from build123d import *

# Parameters (mm, degrees)
F0_W      = 23.4
F0_H      = 7.4
F1_DEPTH  = 3.95
F2_R      = 3.69999
F3_R      = 2.499
F4_DEPTH  = 25
F3_R_2    = 3
F5_DEPTH  = 1
F6_R      = 3
F6_R_2    = 2.499
F7_DEPTH  = 1
F8_R      = 3
F9_DEPTH  = 0.5
F10_R     = 3
F11_DEPTH = 0.5


# Not quite as in the source:
# - a fillet or chamfer is up to 0.001 mm smaller than in the source, because OpenCascade refuses the exact size


with BuildPart() as f1:
    # F0 (on Front) → F1 (new body, symmetric)
    with BuildSketch(Plane.XZ):
        Rectangle(F0_W, F0_H)
        with BuildLine():
            ThreePointArc((-7.199, -2.3313088598), (-8.099, -2.499), (-8.999, -2.3313088598))
            Line((-8.999, -2.3313088598), (-8.999, -0.9))
            Line((-8.999, -0.9), (-10.4303088598, -0.9))
            ThreePointArc((-10.4303088598, -0.9), (-10.598, 0), (-10.4303088598, 0.9))
            Line((-10.4303088598, 0.9), (-8.999, 0.9))
            Line((-8.999, 0.9), (-8.999, 2.3313088598))
            ThreePointArc((-8.999, 2.3313088598), (-8.099, 2.499), (-7.199, 2.3313088598))
            Line((-7.199, 2.3313088598), (-7.199, 0.9))
            Line((-7.199, 0.9), (-5.7676911402, 0.9))
            ThreePointArc((-5.7676911402, 0.9), (-5.6, 0), (-5.7676911402, -0.9))
            Line((-5.7676911402, -0.9), (-7.199, -0.9))
            Line((-7.199, -0.9), (-7.199, -2.3313088598))
        make_face(mode=Mode.SUBTRACT)
        with BuildLine():
            Line((7.199, 0.9), (7.199, 2.3313088598))
            ThreePointArc((7.199, 2.3313088598), (8.099, 2.499), (8.999, 2.3313088598))
            Line((8.999, 2.3313088598), (8.999, 0.9))
            Line((8.999, 0.9), (10.4303088598, 0.9))
            ThreePointArc((10.4303088598, 0.9), (10.598, 0), (10.4303088598, -0.9))
            Line((10.4303088598, -0.9), (8.999, -0.9))
            Line((8.999, -0.9), (8.999, -2.3313088598))
            ThreePointArc((8.999, -2.3313088598), (8.099, -2.499), (7.199, -2.3313088598))
            Line((7.199, -2.3313088598), (7.199, -0.9))
            Line((7.199, -0.9), (5.7676911402, -0.9))
            ThreePointArc((5.7676911402, -0.9), (5.6, 0), (5.7676911402, 0.9))
            Line((5.7676911402, 0.9), (7.199, 0.9))
        make_face(mode=Mode.SUBTRACT)
    extrude(amount=F1_DEPTH, both=True)

    # F2 (radius 3.7 in the source; OpenCascade refuses exactly that, so slightly less here)
    f2_edges = [f1.edges().sort_by_distance(p)[0] for p in [
        (-11.7, 0, -3.7),
        (-11.7, 0, 3.7),
        (11.7, 0, 3.7),
        (11.7, 0, -3.7),
    ]]
    fillet(f2_edges, radius=F2_R)

    # F3 (on face) → F4 (cut)
    with BuildSketch(Plane.XY.offset(3.7)):
        Circle(F3_R)
    extrude(amount=-F4_DEPTH, mode=Mode.SUBTRACT)

    # F3 (on face) → F5 (cut)
    with BuildSketch(Plane.XY.offset(3.7)):
        Circle(F3_R_2)
        Circle(F3_R, mode=Mode.SUBTRACT)
    extrude(amount=-F5_DEPTH, mode=Mode.SUBTRACT)

    # F6 (on face) → F7 (cut)
    with BuildSketch(Plane(origin=(0, 0, -3.7), x_dir=(1, 0, 0), z_dir=(0, 0, -1))):
        Circle(F6_R)
        Circle(F6_R_2, mode=Mode.SUBTRACT)
    extrude(amount=-F7_DEPTH, mode=Mode.SUBTRACT)

    # F8 (on face) → F9 (cut)
    with BuildSketch(Plane.XZ.offset(3.95)):
        with Locations((-8, 0)):
            Circle(F8_R)
        with Locations((8.099, 0)):
            Circle(F8_R)
    extrude(amount=-F9_DEPTH, mode=Mode.SUBTRACT)

    # F10 (on face) → F11 (cut)
    with BuildSketch(Plane(origin=(0, 3.95, 0), x_dir=(-1, 0, 0), z_dir=(0, 1, 0))):
        with Locations((-8, 0)):
            Circle(F10_R)
        with Locations((8.099, 0)):
            Circle(F10_R)
    extrude(amount=-F11_DEPTH, mode=Mode.SUBTRACT)


solid = f1.part
Verification items for the finished model (mm, model axes). A direction names the side the tool comes from. Give positions to 0.01 mm unless a question says otherwise; leave off trailing zeros. Order: outer loops, then holes, each group sorted by start corner. A loop starts at its lowest first (then second) coordinate and runs counter-clockwise, first axis right, second up. Notation, with made-up numbers: (-27, -14.75) -> (-16, -14.75) arc R22 ccw to (-16, 8.25) -> close; hole circle Ø10 at (-32, 87). An arc over 180 degrees is marked (long way). Answer as CSV lines item,"result".
Q1. Release check for a two-part mould opening along Y. For faces 4 (the flat face through (-2, 2, 2.7)), 5 (the flat face through (6, 0, -0.9)), 6 (the flat face through (9.4, -3.45, -1.3)), 7 (the cylindrical face through (-3, 0, 3)) record: +Y half, -Y half, draft (parallel to the pull), parting line (faces both ways), or undercut.
Solutions:
face 4,"undercut"
face 5,"draft"
face 6,"-Y half"
face 7,"undercut"
Q2. Sectioned sample at B-B on x = 0. Record the cut outline in (y, z), plus the area to 3 significant figures.
Solutions:
outline,"(-3.95, -3.7) -> (-3, -3.7) -> (-3, -2.7) -> (-2.5, -2.7) -> (-2.5, 2.7) -> (-3, 2.7) -> (-3, 3.7) -> (-3.95, 3.7) -> close; (2.5, -2.7) -> (3, -2.7) -> (3, -3.7) -> (3.95, -3.7) -> (3.95, 3.7) -> (3, 3.7) -> (3, 2.7) -> (2.5, 2.7) -> close"
area,"19.5 mm²"
Q3. Depth check by flat-ended pin: pin 1 (3 mm diameter, centred on y = 2, z = -2, fed in from -X); pin 2 (0.7 mm diameter, centred on y = 1, z = -1.5, fed in from +X); pin 3 (4 mm diameter, centred on x = 0, y = 0, fed in from -Z); pin 4 (4 mm diameter, centred on y = 2.5, z = -3, fed in from +X). Enter the tip coordinate at first touch or a pass-through.
Solutions:
pin 1,"stops at x = -11.67"
pin 2,"stops at x = 11.52"
pin 3,"passes through"
pin 4,"stops at x = 11.56"
Q4. Scan lines: probe 1 along X at (y, z) = (0, 1.15); probe 2 along X at (y, z) = (-2, 2); probe 3 along Z at (x, y) = (-8, -3.75). Record each from-to range of solid material in increasing order.
Solutions:
probe 1,"x = -11.52 to -9, -7.2 to -2.5, 2.5 to 7.2, 9 to 11.52"
probe 2,"x = -11.11 to -9, -7.2 to -1.5, 1.5 to 7.2, 9 to 11.11"
probe 3,"z = -3.7 to -3, 3 to 3.7"
Q5. Sectioned sample at A-A on z = -1.75. Count the separate pieces of the cut face and the enclosed holes in it, plus the area to 3 significant figures.
Solutions:
separate pieces,"3"
enclosed holes,"1"
area,"124 mm²"
Q6. Sectioned sample at D-D on x = 8.5. Record the cut outline in (y, z), plus the area to 3 significant figures.
Solutions:
outline,"(-3.95, -3.67) -> (3.95, -3.67) -> (3.95, -2.96) -> (3.45, -2.96) -> (3.45, -2.47) -> (-3.45, -2.47) -> (-3.45, -2.97) -> (-3.95, -2.97) -> close; (-3.95, 2.97) -> (-3.45, 2.97) -> (-3.45, 2.47) -> (3.45, 2.47) -> (3.45, 2.96) -> (3.95, 2.96) -> (3.95, 3.67) -> (-3.95, 3.67) -> close"
area,"18.0 mm²"
Q7. Access from +Z, -Z, +X, -X, +Y, -Y to the whole of each face (thin tool, end or side, straight path). Record for faces 1 (the flat face through (-6, 0, 0.9)), 2 (the cylindrical face through (-3, 0, -3)), 3 (the cylindrical face through (-10.87, 3.7, -1.15)).
Solutions:
face 1,"+Y, -Y"
face 2,"-Z"
face 3,"+Y"
